CAD build for the part. Positions are in the model's coordinates, mm. A direction names the side the tool comes from. Give positions to 0.01 mm unless a question says otherwise; leave off trailing zeros. Order: outer loops, then holes, each group sorted by start corner. A loop starts at its lowest first (then second) coordinate and runs counter-clockwise, first axis right, second up.
```python
from build123d import *

# Parameters (mm, degrees)
F0_R     = 33
F0_R_2   = 26.5
F1_DEPTH = 5
F0_R_3   = 17
F2_DEPTH = 80
F3_W     = 4.817946
F3_H     = 30
F3_W_2   = 5.182054
F4_DEPTH = 50


with BuildPart() as f1:
    # F0 (on Top) → F1 (new body)
    with BuildSketch(Plane.XY):
        Circle(F0_R)
        Circle(F0_R_2, mode=Mode.SUBTRACT)
    extrude(amount=-F1_DEPTH)

    # F0 (on Top) → F2 (join)
    with BuildSketch(Plane.XY):
        Circle(F0_R_2)
        Circle(F0_R_3, mode=Mode.SUBTRACT)
    extrude(amount=-F2_DEPTH)

    # F3 (on Front) → F4 (cut, symmetric)
    with BuildSketch(Plane.XZ):
        with Locations((2.408973, -32)):
            Rectangle(F3_W, F3_H)
        with Locations((-2.591027, -32)):
            Rectangle(F3_W_2, F3_H)
    extrude(amount=F4_DEPTH, both=True, mode=Mode.SUBTRACT)


solid = f1.part
```
Item 1: Slice it at C-C (z = -46). Give the cut face in (x, y), and give its area (3 significant figures).
Item 2: Slice it at D-D (x = 13). Give the cut face in (y, z).
Item 3: Tool access for faces 1 (the face through (30.5, -12.6, -2.5)), 2 (the face through (0, 27, -5)), 3 (the face through (-5.182, -21, -32)): list every direction of +Z, -Z, +X, -X, +Y, -Y with a clear straight run to the whole face (end or side of a thin tool).
Item 4: Slice it at B-B (x = 0). Give the cut face in (y, z).
Item 5: Slice it at A-A (y = 0). Give the cut face in (x, z), and give its area (4 significant figures).
Item 6: Wall check: L1, parallel to Y at x = 0, z = -56; L2, parallel to Z at x = -11, y = 28.5; L3, parallel to X at y = 9, z = -56. Give the ranges that are in metal, low to high.
Item 7: Drop flat-ended pins along their axis: pin 1 Ø6 at (y, z) = (-25, -20.5) entering from -X; pin 2 Ø5 at (y, z) = (19, -28.5) entering from -X; pin 3 Ø1.5 at (x, z) = (15, -63) entering from +Y; pin 4 Ø5 at (x, y) = (-0.5, -23.5) entering from +Z. Give the stop position or say it passes through.
Item 8: Two-plate mould, pull along Y, no slides. Class faces 4 (the face through (-0.4, -17.3, -80)), 5 (the face through (-5.74, -25.87, -41.98)), 6 (the face through (16.215, 5.106, -39.44)): released by +Y, released by -Y, zero draft, split by the parting line, or undercut.
A:
1. outline: (-5.18, -25.99) - (-5.18, -16.19) arc R17 cw to (-5.18, 16.19) - (-5.18, 25.99) arc R26.5 ccw to start; (4.82, -26.06) arc R26.5 ccw to (4.82, 26.06) - (4.82, 16.3) arc R17 cw to (4.82, -16.3) - close
1. area: 1,110 mm2
2. outline: (-30.33, -5) - (-23.09, -5) - (-23.09, -80) - (-10.95, -80) - (-10.95, 0) - (-30.33, 0) - close; (10.95, -80) - (23.09, -80) - (23.09, -5) - (30.33, -5) - (30.33, 0) - (10.95, 0) - close
3. face 1: +Z, -Z
3. face 2: -Z
3. face 3: +Y, -Y
4. outline: (-33, -5) - (-26.5, -5) - (-26.5, -17) - (-17, -17) - (-17, 0) - (-33, 0) - close; (-26.5, -80) - (-17, -80) - (-17, -47) - (-26.5, -47) - close; (17, -80) - (26.5, -80) - (26.5, -47) - (17, -47) - close; (17, -17) - (26.5, -17) - (26.5, -5) - (33, -5) - (33, 0) - (17, 0) - close
5. outline: (-33, -5) - (-26.5, -5) - (-26.5, -80) - (-17, -80) - (-17, 0) - (-33, 0) - close; (17, -80) - (26.5, -80) - (26.5, -5) - (33, -5) - (33, 0) - (17, 0) - close
5. area: 1,585 mm2
6. L1: y = -26.5 to -17, 17 to 26.5
6. L2: z = -5 to 0
6. L3: x = -24.92 to -14.42, 14.42 to 24.92
7. pin 1: stops at x = -14.77
7. pin 2: stops at x = -20.74
7. pin 3: stops at y = 22.34
7. pin 4: stops at z = 0
8. face 4: zero draft
8. face 5: split by the parting line
8. face 6: undercut
